Here's the drawing with two shaded views (mm, measured from the low corner). I have some questions. A direction names the side the tool comes from. Give positions to 0.01 mm unless a question says otherwise; leave off trailing zeros. Loops run counter-clockwise (first coordinate to the right, second up) from the corner with the lowest first, then second, coordinate; pieces in that order, holes last. Notation, with made-up numbers: M -1.75,82.5 L 38.25,82.5 A23 cw 38.25,101.5 Z; hole C 78.25,-37.5 d2. An arc over 180 degrees is marked long. Write item = value, one per line. Start each with the question number.
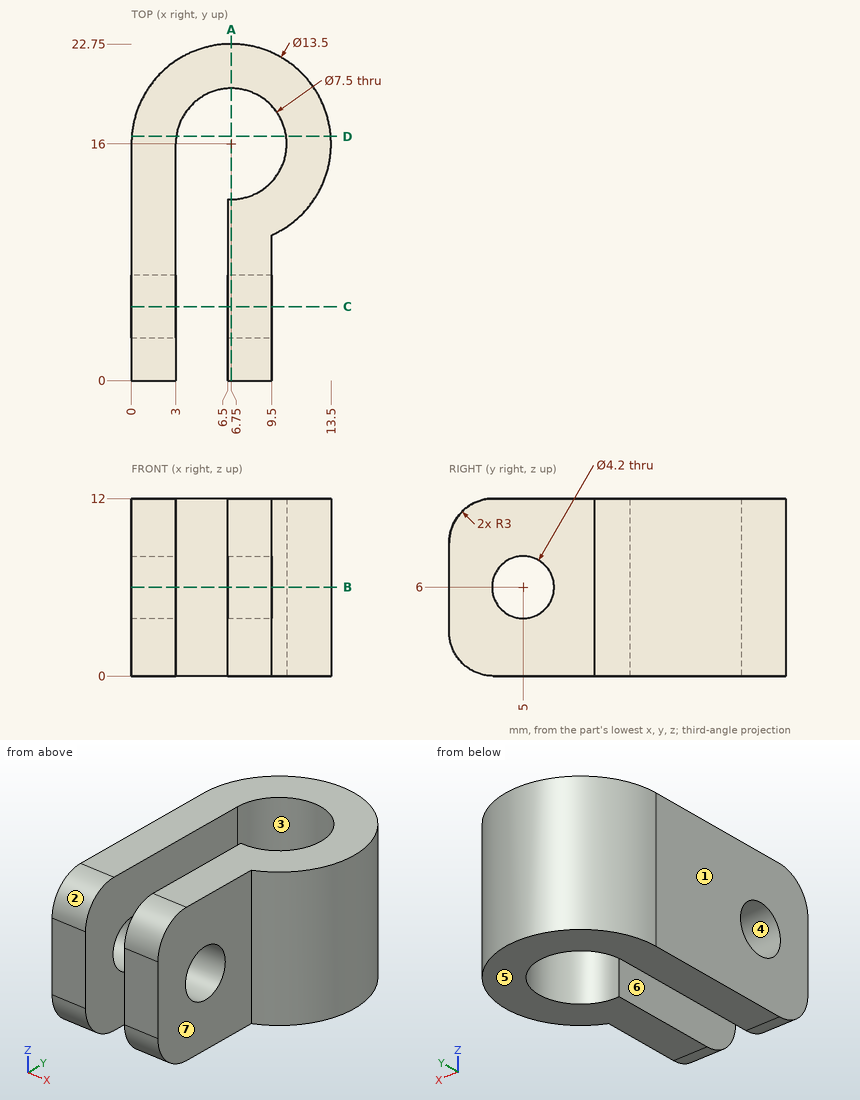
Q1. If we section it at D-D, the plane y = 16.5: List the corners of the cut face in (x, z) for me, then the cut area to 3 significant figures.
Q2. On a 3-axis mill with a long thin cutter (end or side, diameter ignored), from which of +Z, -Z, +X, -X, +Y, -Y can I reach the whole of each face in a straight line? I mean the marked faces 5, 6 and 7. Say none if no direction works.
Q3. We'd pull the mould along Y, two halves only. Please class the marked faces 1, 2, 3 and 4: pulls with the +Y half, pulls with the -Y half, needs draft (parallel to the pull), parting line crosses it, or undercut.
Q4. If we section it at A-A, the plane x = 6.75: List the corners of the cut face in (y, z) for me, then the cut area to 3 significant figures.
Q5. If I drill on line 1 along Z through (x, y) = (1.8, 5); line 2 along X through (y, z) = (3.5, 10.5); line 3 along X through (y, z) = (12.75, 5.75), over which ranges is the centre line in solid material (lowest first)?
Q6. Will these pins go through, and if not, where does the flat tip stop? pin 1 (1.5 mm diameter, centred on x = 11.5, z = 5, fed in from -Y); pin 2 (3 mm diameter, centred on y = 7.5, z = 8.5, fed in from +X); pin 3 (3.5 mm diameter, centred on y = 5, z = 6, fed in from +X).
Q7. If we section it at B-B, the plane z = 6: List the corners of the cut face in (x, y) for me, then the cut area to 3 significant figures.
Q8. If we section it at C-C, the plane y = 5: List the corners of the cut face in (x, z) for me, then the cut area to 3 significant figures.
Resolved:
q1.outline = M 0.02,0 L 3.03,0 L 3.03,12 L 0.02,12 Z; M 10.47,0 L 13.48,0 L 13.48,12 L 10.47,12 Z
q1.area = 72.4 mm²
q2.face_5 = -Z, +X, -X, +Y, -Y
q2.face_6 = +Z, -Z, -Y
q2.face_7 = +Z, -Z, +X, -Y
q3.face_1 = needs draft
q3.face_2 = pulls with the -Y half
q3.face_3 = undercut
q3.face_4 = undercut
q4.outline = M 0,3 A3 ccw 3,0 L 12.25,0 L 12.25,12 L 3,12 A3 ccw 0,9 Z; M 19.75,0 L 22.75,0 L 22.75,12 L 19.75,12 Z; hole C 5,6 d4.2
q4.area = 165 mm²
q5.line_1 = 0 to 3.9, 8.1 to 12
q5.line_2 = 0 to 3, 6.5 to 9.5
q5.line_3 = 0 to 3, 8.62 to 12.67
q6.pin_1 = 10.56
q6.pin_2 = 9.5
q6.pin_3 = through
q7.outline = M 0,0 L 3,0 L 3,2.9 L 0,2.9 Z; M 0,7.1 L 3,7.1 L 3,16 A3.75 cw long 6.5,12.26 L 6.5,7.1 L 9.5,7.1 L 9.5,9.84 A6.75 ccw long 0,16 Z; M 6.5,0 L 9.5,0 L 9.5,2.9 L 6.5,2.9 Z
q7.area = 126 mm²
q8.outline = M 0,0 L 3,0 L 3,3.9 L 0,3.9 Z; M 0,8.1 L 3,8.1 L 3,12 L 0,12 Z; M 6.5,0 L 9.5,0 L 9.5,3.9 L 6.5,3.9 Z; M 6.5,8.1 L 9.5,8.1 L 9.5,12 L 6.5,12 Z
q8.area = 46.8 mm²
